Design review of the part built by this model. Coordinates are the model's own, in mm. A direction names the side the tool comes from. Round coordinates to 2 decimals unless told otherwise and drop trailing zeros. Loops run counter-clockwise (first coordinate to the right, second up) from the corner with the lowest first, then second, coordinate; pieces in that order, holes last. Notation, with made-up numbers: (-21, -23.75) -> (19, -23.75) arc R21 cw to (19, 10.25) -> close; hole circle Ø1 at (-35.5, 54.5). An arc over 180 degrees is marked (long way). Write each question's results on one line, items separated by ' | '. Start each with the question number.
from build123d import *

# Parameters (mm, degrees)
F1_DEPTH = 100
F3_DEPTH = 5
F5_DEPTH = 5


with BuildPart() as f1:
    # F0 (on Front) → F1 (new body)
    with BuildSketch(Plane.XZ):
        with BuildLine():
            Line((-53.263988, 129.954544), (-58.263987, 129.954544))
            Line((-58.263987, 129.954544), (-58.263987, -18.045456))
            ThreePointArc((-58.263987, -18.045456), (-57.678201, -19.459669), (-56.263987, -20.045456))
            Line((-56.263987, -20.045456), (34.736013, -20.045456))
            ThreePointArc((34.736013, -20.045456), (36.150226, -19.459669), (36.736013, -18.045456))
            Line((36.736013, -18.045456), (36.736013, 129.954544))
            Line((36.736013, 129.954544), (31.736013, 129.954544))
            Line((31.736013, 129.954544), (31.736013, -13.045456))
            ThreePointArc((31.736013, -13.045456), (31.150226, -14.459669), (29.736013, -15.045456))
            Line((29.736013, -15.045456), (-51.263988, -15.045456))
            ThreePointArc((-51.263988, -15.045456), (-52.678202, -14.459669), (-53.263988, -13.045456))
            Line((-53.263988, -13.045456), (-53.263988, 129.954544))
        make_face()
    extrude(amount=F1_DEPTH)

    # F2 (on face) → F3 (cut)
    with BuildSketch(Plane.YZ.offset(36.736013)):
        with BuildLine():
            ThreePointArc((-20, 79.954544), (-71.213203, 101.167748), (-50, 49.954544))
            ThreePointArc((-50, 49.954544), (-28.786797, 58.741341), (-20, 79.954544))
        make_face()
    extrude(amount=-F3_DEPTH, mode=Mode.SUBTRACT)

    # F4 (on face) → F5 (cut)
    with BuildSketch(Plane(origin=(-58.263987, 0, 0), x_dir=(0, -1, 0), z_dir=(-1, 0, 0))):
        with BuildLine():
            ThreePointArc((75, 79.954544), (32.32233, 97.632214), (50, 54.954544))
            ThreePointArc((50, 54.954544), (67.67767, 62.276875), (75, 79.954544))
        make_face()
    extrude(amount=-F5_DEPTH, mode=Mode.SUBTRACT)


solid = f1.part
1) Take a section at A-A (z = 37). Write out the cut boundary in (x, y), plus the area to 4 significant figures.
2) Take a section at D-D (z = 76). Write out the cut boundary in (x, y), plus the area to 3 significant figures.
3) Insertion check: pin 1 (4 mm diameter, centred on y = -24, z = 87, fed in from +X); pin 2 (5 mm diameter, centred on x = 11, y = -81.5, fed in from +Z). Each pin has a flat end and moves straight along its axis. Give the tip position at first contact, or say it passes through.
4) Take a section at B-B (y = -28.5). Write out the cut boundary in (x, z).
5) For faces 1 (the face through (-10, -49, -15.045)), 2 (the face through (34, -49, 129.955)), list the 3-axis set-ups (+Z, -Z, +X, -X, +Y, -Y) from which the entire face can be reached by the end or side of a thin tool; tool diameter is ignored.
6) The part is to be moulded in two halves that separate along X. For faces 3 (the face through (-53.264, -38, 57)), 4 (the face through (31.736, -49, 44)), 5 (the face through (-57, 0, 33)), 6 (the face through (36.736, -49, 38)), say which applies: +X half, -X half, draft (parallel to the pull), parting line (faces both ways), or undercut.
7) Take a section at C-C (y = -6.5). Write out the cut boundary in (x, z).
8) To check wall thickness, follow line 1 (Z direction, x = -56.75, y = -50); line 2 (Z direction, x = 35, y = -50); line 3 (X direction, y = -58.5, z = 41). State the ranges of each line that lie inside material, in increasing order. Write a range as from..to.
Geometry check:
1) outline: (-58.26, -100) -> (-53.26, -100) -> (-53.26, 0) -> (-58.26, 0) -> close; (31.74, -100) -> (36.74, -100) -> (36.74, 0) -> (31.74, 0) -> close | area: 1,000 mm^2
2) outline: (-58.26, -100) -> (-53.26, -100) -> (-53.26, -74.69) -> (-58.26, -74.69) -> close; (-58.26, -25.31) -> (-53.26, -25.31) -> (-53.26, 0) -> (-58.26, 0) -> close; (31.74, -100) -> (36.74, -100) -> (36.74, -79.74) -> (31.74, -79.74) -> close; (31.74, -20.26) -> (36.74, -20.26) -> (36.74, 0) -> (31.74, 0) -> close | area: 456 mm^2
3) pin 1: stops at x = -53.26 | pin 2: stops at z = -15.05
4) outline: (-58.26, -18.05) arc R2 ccw to (-56.26, -20.05) -> (34.74, -20.05) arc R2 ccw to (36.74, -18.05) -> (36.74, 59.03) -> (31.74, 59.03) -> (31.74, -13.05) arc R2 cw to (29.74, -15.05) -> (-51.26, -15.05) arc R2 cw to (-53.26, -13.05) -> (-53.26, 67.2) -> (-58.26, 67.2) -> close; (-58.26, 92.71) -> (-53.26, 92.71) -> (-53.26, 129.95) -> (-58.26, 129.95) -> close; (31.74, 100.88) -> (36.74, 100.88) -> (36.74, 129.95) -> (31.74, 129.95) -> close
5) face 1: +Z, +Y, -Y | face 2: +Z, +X, -X, +Y, -Y
6) face 3: undercut | face 4: undercut | face 5: draft | face 6: +X half
7) outline: (-58.26, -18.05) arc R2 ccw to (-56.26, -20.05) -> (34.74, -20.05) arc R2 ccw to (36.74, -18.05) -> (36.74, 129.95) -> (31.74, 129.95) -> (31.74, -13.05) arc R2 cw to (29.74, -15.05) -> (-51.26, -15.05) arc R2 cw to (-53.26, -13.05) -> (-53.26, 129.95) -> (-58.26, 129.95) -> close
8) line 1: z = -19.99..54.95, 104.95..129.95 | line 2: z = -20.03..49.95, 109.95..129.95 | line 3: x = -58.26..-53.26, 31.74..36.74
